Part model, mm, in its own coordinate system. Face numbers are marked on the shaded views. A direction names the side the tool comes from. Coordinates: 2 decimals unless noted, no trailing zeros. Write each loop counter-clockwise with the first axis right and the second up, starting at its lowest first coordinate (ties: lowest second). Pieces come first, ordered by that corner, then holes. Notation, with made-up numbers: (24, -11.5) -> (28, -11.5) arc R24 cw to (28, 8.5) -> close; hole circle Ø2 at (-21, 70.25). An arc over 180 degrees is marked (long way). Write item = value, one per line. Start each with the question number.
Q1. Band-saw the part on C-C, the plane z = 4.5. List the corners of the cut face in (x, y), plus the area to 3 significant figures.
Q2. Tool access for the marked faces 4, 5, 6 and 7: list every direction of +Z, -Z, +X, -X, +Y, -Y with a clear straight run to the whole face (end or side of a thin tool).
Q3. Band-saw the part on D-D, the plane z = 1.75. List the corners of the cut face in (x, y), plus the area to 3 significant figures.
Q4. Band-saw the part on A-A, the plane x = -20.1. List the corners of the cut face in (y, z), plus the area to 3 significant figures.
Q5. Probe line 1 (X direction, y = 4.55, z = 4); line 2 (X direction, y = 7.25, z = 0.5); line 3 (Z direction, x = 20.1, y = 3.05). List the from-to ranges inside material, lowest first.
Q6. Band-saw the part on B-B, the plane y = 11. List the corners of the cut face in (x, z), plus the area to 3 significant figures.
Q7. Pull direction X, two halves, no side cores. Call the marked faces 1, 2 and 3: released by +X, released by -X, zero draft, split by the parting line, or undercut.
Q8. Pin check, flat tips, straight feed: P1, Ø1.9, axis at x = -20.1, z = 4, coming from the -Y side; P2, Ø2.5, axis at x = -20.5, z = 4.5, coming from the +Y side; P3, Ø3, axis at y = 12.5, z = 7, coming from the +X side; P4, Ø4, axis at y = 24.5, z = 4, coming from the +X side. Stop position of each tip, or through.
Autodesk Fusion 360 part; units mm, degrees
sketch "Sketch1" plane through (0, 0, 0) normal (0, 0, 1) x (1, 0, 0)
  line L0 (0, 0) -> (0, 25.1) construction
  line L1 (-28.1, 2.5) -> (-12.6, 2.5)
  line L2 (-12.6, 2.5) -> (-12.6, 12.6)
  line L3 (-16.3497, 12.6) -> (-28.1, 12.6)
  line L4 (-28.1, 12.6) -> (-28.1, 2.5)
  line L5 (28.1, 12.6) -> (28.1, 2.5)
  line L6 (16.3497, 12.6) -> (28.1, 12.6)
  line L7 (28.1, 2.5) -> (12.6, 2.5)
  line L8 (12.6, 2.5) -> (12.6, 12.6)
  arc A0 (16.3497, 12.6) -> (-16.3497, 12.6) centre (0, 12.5) ccw
  arc A1 (12.6, 12.5) -> (-12.6, 12.5) centre (0, 12.5) ccw
  line L9 (-28.1, 12.6) -> (-16.35, 12.6)
  line L10 (-16.35, 12.6) -> (-16.35, 6.25)
  line L11 (-16.35, 6.25) -> (-28.1, 6.25)
  line L12 (-28.1, 6.25) -> (-28.1, 12.6)
  line L13 (28.1, 12.6) -> (16.35, 12.6)
  line L14 (16.35, 6.25) -> (28.1, 6.25)
  line L15 (16.35, 12.6) -> (16.35, 6.25)
  point P0 (0, 12.5)
  point P1 (-12.6, 12.6)
  point P2 (-28.1, 2.5)
  point P3 (12.6, 12.6)
  point P4 (-28.1, 2.5)
  point P5 (-20.1, 6.15)
  point P6 (-16.35, 12.5)
  point P7 (20.1, 6.15)
  dimension "d1" = 25.2
  dimension "d2" = 32.7
  dimension "d3" = 11.75
  dimension "d4" = 6.35
extrude "Extrude1" add sketch "Sketch1" along normal blind 8 contours L1 L2 L4 L5 L7 L8 A0 A1 L10 L11 L14 L15
sketch "Sketch2" plane through (0, 6.25, 0) normal (0, 1, 0) x (-1, 0, 0)
  line L0 (16.35, 0) -> (28.1, 0)
  line L1 (28.1, 0) -> (28.1, 8)
  line L2 (28.1, 8) -> (16.35, 8)
  line L3 (16.35, 8) -> (16.35, 0)
  line L4 (0, 8) -> (0, 0) construction
  point P0 (20.1, 4)
  point P1 (-20.1, 4)
hole "Hole1" at (-20.1, 6.25, 4) at (20.1, 6.25, 4) direction (0, -1, 0) diameter 3.2 end through all counterbore diameter 6 counterbore depth 3
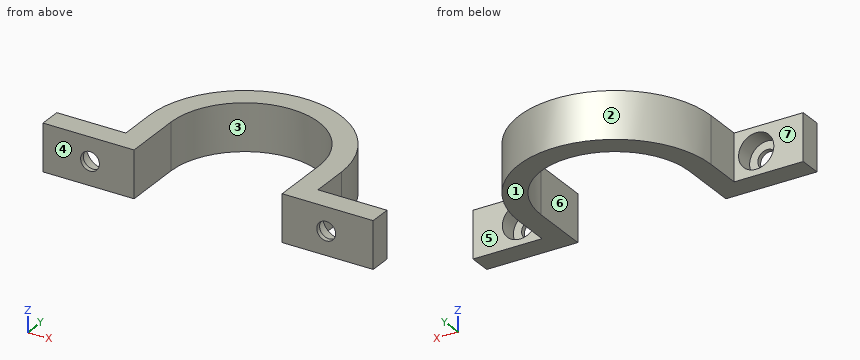
Ans:
q1.outline = (-28.1, 2.5) -> (-21.62, 2.5) -> (-21.62, 3.25) -> (-23.06, 3.25) -> (-23.06, 6.25) -> (-28.1, 6.25) -> close; (-18.58, 2.5) -> (-12.6, 2.5) -> (-12.6, 12.6) arc R12.6 cw to (12.6, 12.6) -> (12.6, 2.5) -> (18.58, 2.5) -> (18.58, 3.25) -> (17.14, 3.25) -> (17.14, 6.25) -> (16.35, 6.25) -> (16.35, 12.6) arc R16.35 ccw to (-16.35, 12.6) -> (-16.35, 6.25) -> (-17.14, 6.25) -> (-17.14, 3.25) -> (-18.58, 3.25) -> close; (21.62, 2.5) -> (28.1, 2.5) -> (28.1, 6.25) -> (23.06, 6.25) -> (23.06, 3.25) -> (21.62, 3.25) -> close
q1.area = 294 mm2
q2.face_4 = +Z, -Z, +X, -X, -Y
q2.face_5 = +Z, -Z, +X, +Y
q2.face_6 = +Z, -Z, -Y
q2.face_7 = +Z, -Z, -X, +Y
q3.outline = (-28.1, 2.5) -> (-12.6, 2.5) -> (-12.6, 12.6) arc R12.6 cw to (12.6, 12.6) -> (12.6, 2.5) -> (28.1, 2.5) -> (28.1, 6.25) -> (22.08, 6.25) -> (22.08, 3.25) -> (18.12, 3.25) -> (18.12, 6.25) -> (16.35, 6.25) -> (16.35, 12.6) arc R16.35 ccw to (-16.35, 12.6) -> (-16.35, 6.25) -> (-18.12, 6.25) -> (-18.12, 3.25) -> (-22.08, 3.25) -> (-22.08, 6.25) -> (-28.1, 6.25) -> close
q3.area = 310 mm2
q4.outline = (2.5, 0) -> (6.25, 0) -> (6.25, 1) -> (3.25, 1) -> (3.25, 2.4) -> (2.5, 2.4) -> close; (2.5, 5.6) -> (3.25, 5.6) -> (3.25, 7) -> (6.25, 7) -> (6.25, 8) -> (2.5, 8) -> close
q4.area = 9.60 mm2
q5.line_1 = -28.1 to -23.1, -17.1 to -12.6, 12.6 to 17.1, 23.1 to 28.1
q5.line_2 = -16.35 to -12.6, 12.6 to 16.35
q5.line_3 = 0 to 2.4, 5.6 to 8
q6.outline = (-16.35, 0) -> (-12.6, 0) -> (-12.6, 8) -> (-16.35, 8) -> close; (12.6, 0) -> (16.35, 0) -> (16.35, 8) -> (12.6, 8) -> close
q6.area = 60.0 mm2
q7.face_1 = zero draft
q7.face_2 = split by the parting line
q7.face_3 = undercut
q8.P1 = through
q8.P2 = 3.25
q8.P3 = 16.35
q8.P4 = 12.94
